Input: part model. Units: mm. Frame: model coordinates. Face numbers are marked on the shaded views. A direction names the side the tool comes from. Give positions to 0.01 mm unless a question says otherwise; leave off trailing zeros. Write each loop counter-clockwise with the first axis right and the second up, starting at its lowest first coordinate (ties: lowest second). Pieces come first, ordered by that corner, then holes. Notation, with made-up numbers: (4, -9.75) -> (57, -9.75) arc R35 cw to (57, 29.25) -> close; hole circle Ø3 at (1, 52.25). An arc over 180 degrees is marked (long way). Answer as a JSON object with one key per item and string values. Group by question number.
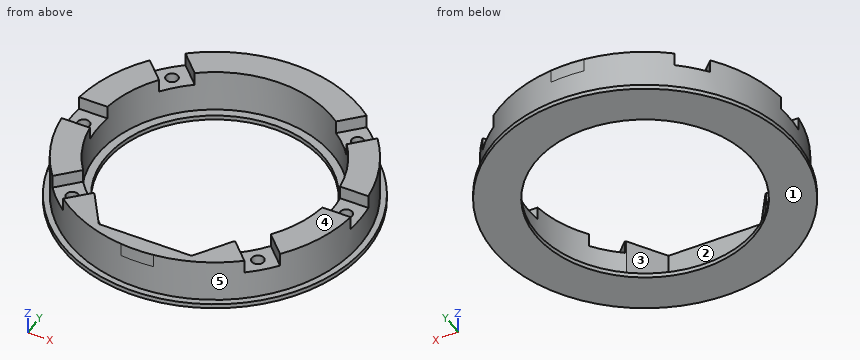
Autodesk Inventor part; units mm, degrees
ref_plane "YZ Plane" through (0, 0, 0) normal (1, 0, 0) x (0, 1, 0)
ref_plane "XZ Plane" through (0, 0, 0) normal (0, 1, 0) x (-1, 0, 0)
ref_plane "XY Plane" through (0, 0, 0) normal (0, 0, 1) x (1, 0, 0)
sketch "Skizze1" plane through (0, 0, 0) normal (0, 0, 1) x (1, 0, 0)
  circle A0 centre (0, 0) radius 18
  circle A1 centre (0, 0) radius 25
  dimension "d0" = 36
  dimension "d1" = 50
extrude "Extrusion1" add sketch "Skizze1" along normal blind 35
sketch "Skizze2" plane through (0, 0, 35) normal (0, 0, 1) x (1, 0, 0)
  circle A0 centre (0, 0) radius 19.3
  line L0 (0, -19.3) -> (0, -21.4)
  line L1 (0, -21.4) -> (-7.65, -21.4)
  line L2 (-7.65, -21.4) -> (7.65, -21.4)
  line L3 (7.65, -21.4) -> (7.65, -17.7191)
  line L4 (-7.65, -21.4) -> (-7.65, -17.7191)
  circle A1 centre (0, 0) radius 25
  circle A2 centre (0, 0) radius 18
  circle A3 centre (0, 0) radius 25
  circle A4 centre (0, 0) radius 18
  circle A5 centre (0, 0) radius 19.3
  dimension "d4" = 38.6
  dimension "d5" = 2.1
  dimension "d6" = 7.65
  dimension "d7" = 90
  dimension "d8" = 15.3
extrude "Extrusion2" cut sketch "Skizze2" against normal blind 34 contours A0 | A0 L0 L1 L4 | L3 L2 L0 A0 | A2
fillet "Rundung1" radius 4 2 edges at (-7.65, -17.7191, 18) (7.65, -17.7191, 18)
sketch "Skizze3" plane through (0, 0, 35) normal (0, 0, 1) x (1, 0, 0)
  arc A0 (9.65, -16.7143) -> (7.65, -20.1784) centre (11.65, -20.1784) ccw
  line L0 (7.65, -20.1784) -> (7.65, -21.4)
  line L1 (7.65, -21.4) -> (-7.65, -21.4)
  line L2 (-7.65, -21.4) -> (-7.65, -20.1784)
  arc A1 (-7.65, -20.1784) -> (-9.65, -16.7143) centre (-11.65, -20.1784) ccw
  arc A2 (9.65, -16.7143) -> (-9.65, -16.7143) centre (0, 0) ccw
  circle A3 centre (0, 0) radius 25
extrude "Extrusion3" cut sketch "Skizze3" against normal blind 25
sketch "Skizze4" plane through (0, 0, 10) normal (0, 0, 1) x (1, 0, 0)
  circle A0 centre (0, 0) radius 24
  circle A1 centre (0, 0) radius 25
  arc A2 (9.65, -16.7143) -> (7.65, -20.1784) centre (11.65, -20.1784) ccw
  line L0 (7.65, -21.4) -> (7.65, -20.1784)
  line L1 (-7.65, -21.4) -> (7.65, -21.4)
  line L2 (-7.65, -20.1784) -> (-7.65, -21.4)
  arc A3 (-7.65, -20.1784) -> (-9.65, -16.7143) centre (-11.65, -20.1784) ccw
  arc A4 (9.65, -16.7143) -> (-9.65, -16.7143) centre (0, 0) ccw
  dimension "d14" = 48
extrude "Extrusion4" cut sketch "Skizze4" against normal blind 9.25 contours A1
sketch "Skizze5" plane through (0, 0, 10) normal (0, 0, 1) x (1, 0, 0)
  circle A0 centre (0, 0) radius 24
  arc A1 (9.65, -16.7143) -> (7.65, -20.1784) centre (11.65, -20.1784) ccw
  line L0 (7.65, -21.4) -> (7.65, -20.1784)
  line L1 (-7.65, -21.4) -> (7.65, -21.4)
  line L2 (-7.65, -20.1784) -> (-7.65, -21.4)
  arc A2 (-7.65, -20.1784) -> (-9.65, -16.7143) centre (-11.65, -20.1784) ccw
  arc A3 (9.65, -16.7143) -> (-9.65, -16.7143) centre (0, 0) ccw
extrude "Extrusion5" cut sketch "Skizze5" against normal blind 2.2
sketch "Skizze6" plane through (0, 0, 7.8) normal (0, 0, 1) x (1, 0, 0)
  line L0 (30, -2.706) -> (-30, -2.706)
  line L1 (-30, -2.706) -> (-30, 2.706)
  line L2 (-30, 2.706) -> (30, 2.706)
  line L3 (30, 2.706) -> (30, -2.706)
  line L4 (30, -2.706) -> (-30, 2.706) construction
  line L5 (-30, -2.706) -> (30, 2.706) construction
  point P0 (0, 0)
  dimension "d33" = 60
extrude "Extrusion6" cut sketch "Skizze6" against normal blind 2.2
sketch "Skizze7" plane through (0, 0, 5.6) normal (0, 0, 1) x (1, 0, 0)
  line L0 (-22.5614, -2.035) -> (-22.5614, 2.035)
  line L1 (-22.5614, 0) -> (-19.3, 0)
  arc A0 (-19.1094, 2.706) -> (-19.1094, -2.706) centre (0, 0) ccw
  line L2 (-19.3, 0) -> (-24, 0)
  circle A1 centre (0, 0) radius 24
  circle A2 centre (-21.65, 0) radius 0.9
  dimension "d34" = 1.8
extrude "Extrusion7" cut sketch "Skizze7" against normal blind 4 contours A2 L1 | L1 A2
mirror "Spiegeln1" about plane through (0, 0, 0) normal (1, 0, 0) of "Extrusion7"
sketch "Skizze8" plane through (0, 0, 7.8) normal (0, 0, 1) x (1, 0, 0)
  point P0 (0, 0)
pattern_circular "Runde Anordnung1" count 8 over 360 about axis through (0, 0, -10) along (0, 0, 1) of "Extrusion7", "Extrusion6"
sketch "Skizze9" plane through (0, -20.9307, 1.6) normal (0, 0, 1) x (1, 0, 0)
  line L0 (-0.8646, -0.4693) -> (0.8646, -0.4693)
  line L1 (-2.706, -0.4693) -> (-0.8646, -0.4693)
  line L2 (-2.706, 40.0401) -> (-2.706, 44.7777)
  line L3 (2.706, 44.7777) -> (2.706, 40.0401)
  arc A0 (2.706, 44.7777) -> (-2.706, 44.7777) centre (0, 20.9307) ccw
  arc A1 (2.706, 40.0401) -> (-2.706, 40.0401) centre (0, 20.9307) ccw
  arc A2 (-2.706, -2.9163) -> (2.706, -2.9163) centre (0, 20.9307) ccw
  line L4 (2.706, -0.4693) -> (2.706, -2.9163)
  line L5 (-2.706, -2.9163) -> (-2.706, -0.4693)
  line L6 (0.8646, -0.4693) -> (2.706, -0.4693)
  arc A3 (-0.8646, -0.4693) -> (0.8646, -0.4693) centre (0, -0.7193) ccw
  arc A4 (-0.8646, -0.4693) -> (0.8646, -0.4693) centre (0, -0.7193) ccw
extrude "Extrusion8" add sketch "Skizze9" along normal blind 4 contours L0 A3
sketch "Skizze10" plane through (-2.706, -21.4, 5.6) normal (0, 0, 1) x (1, 0, 0)
  line L0 (0, 0) -> (5.412, 0)
  line L1 (0, 40.5094) -> (0, 45.247)
  line L2 (5.412, 45.247) -> (5.412, 40.5094)
  arc A0 (5.412, 45.247) -> (0, 45.247) centre (2.706, 21.4) ccw
  arc A1 (5.412, 40.5094) -> (0, 40.5094) centre (2.706, 21.4) ccw
  arc A2 (0, -2.447) -> (5.412, -2.447) centre (2.706, 21.4) ccw
  line L3 (5.412, 0) -> (5.412, -2.447)
  line L4 (0, -2.447) -> (0, 0)
extrude "Extrusion9" add sketch "Skizze10" along normal up to surface (2.2 mm away)
sketch "Skizze11" plane through (0, 0, 7.8) normal (0, 0, 1) x (-0.3826834, -0.9238795, 0)
  line L0 (15.7149, 14.7896) -> (16.8435, 15.2571)
  arc A0 (11.7491, 15.3117) -> (9.8128, 16.6192) centre (0, 0) ccw
  line L1 (16.8435, 15.2571) -> (11.7491, 15.3117)
  line L2 (-18.6903, 4.8128) -> (-23.0673, 6.6258)
  arc A1 (9.8128, -16.6192) -> (16.6192, -9.8128) centre (0, 0) ccw
  line L3 (9.8128, -16.6192) -> (11.6258, -20.9962)
  line L4 (6.6258, -23.0673) -> (4.8128, -18.6903)
  arc A2 (-4.8128, -18.6903) -> (4.8128, -18.6903) centre (0, 0) ccw
  line L5 (-4.8128, -18.6903) -> (-6.6258, -23.0673)
  line L6 (4.8128, 18.6903) -> (6.6258, 23.0673)
  line L7 (20.9962, -11.6258) -> (16.6192, -9.8128)
  line L8 (18.6903, -4.8128) -> (23.0673, -6.6258)
  arc A3 (-9.8128, 16.6192) -> (-16.6192, 9.8128) centre (0, 0) ccw
  line L9 (-9.8128, 16.6192) -> (-11.6258, 20.9962)
  line L10 (-6.6258, 23.0673) -> (-4.8128, 18.6903)
  arc A4 (4.8128, 18.6903) -> (-4.8128, 18.6903) centre (0, 0) ccw
  line L11 (-11.6258, -20.9962) -> (-9.8128, -16.6192)
  line L12 (11.6258, 20.9962) -> (9.8128, 16.6192)
  arc A5 (11.7491, 15.3117) -> (9.8128, 16.6192) centre (0, 0) ccw
  arc A6 (11.7491, 15.3117) -> (15.7149, 14.7896) centre (14.1841, 18.4851) ccw
  line L13 (16.8435, 15.2571) -> (15.7149, 14.7896)
  line L14 (22.6986, 1.1217) -> (16.8435, 15.2571)
  line L15 (21.5699, 0.6543) -> (22.6986, 1.1217)
  arc A7 (21.5699, 0.6543) -> (19.1349, -2.5192) centre (23.1007, -3.0413) ccw
  arc A8 (18.6903, -4.8128) -> (19.1349, -2.5192) centre (0, 0) ccw
  line L16 (-20.9962, 11.6258) -> (-16.6192, 9.8128)
  arc A9 (-6.6258, -23.0673) -> (6.6258, -23.0673) centre (0, 0) ccw
  arc A10 (-18.6903, 4.8128) -> (-9.8128, -16.6192) centre (0, 0) ccw
  arc A11 (-23.0673, 6.6258) -> (-11.6258, -20.9962) centre (0, 0) ccw
  arc A12 (-11.6258, 20.9962) -> (-20.9962, 11.6258) centre (0, 0) ccw
  arc A13 (11.6258, -20.9962) -> (20.9962, -11.6258) centre (0, 0) ccw
  arc A14 (6.6258, 23.0673) -> (-6.6258, 23.0673) centre (0, 0) ccw
  arc A15 (23.0673, -6.6258) -> (11.6258, 20.9962) centre (0, 0) ccw
  point P0 (15.7149, 14.7896)
extrude "Extrusion10" cut sketch "Skizze11" against normal up to surface (6.8 mm away) contours A6 L1 L0
mirror "Spiegeln2" about plane through (0, 0, 0) normal (1, 0, 0) of "Extrusion10"
sketch "Skizze12" plane through (0, 0, 7.8) normal (0, 0, 1) x (-0.3826834, -0.9238795, 0)
  point P0 (0, 0)
sketch "Skizze13" plane through (0, 0, 7.8) normal (0, 0, 1) x (1, 0, 0)
  line L0 (-7.65, -21.4) -> (-9.65, -16.7143)
  arc A0 (-11.5989, -15.4258) -> (-9.65, -16.7143) centre (0, 0) ccw
  line L1 (-11.5989, -15.4258) -> (-14.9489, -18.7758)
  arc A1 (-14.9489, -18.7758) -> (14.9489, -18.7758) centre (0, 0) ccw
  line L2 (14.9489, -18.7758) -> (11.5989, -15.4258)
  arc A2 (9.65, -16.7143) -> (11.5989, -15.4258) centre (0, 0) ccw
  line L3 (9.65, -16.7143) -> (7.65, -21.4)
  line L4 (-7.65, -21.4) -> (7.65, -21.4)
  arc A3 (-11.5989, -15.4258) -> (-9.65, -16.7143) centre (0, 0) ccw
  line L5 (7.65, -21.4) -> (-7.65, -21.4)
  line L6 (-11.5989, -15.4258) -> (-7.65, -21.4)
extrude "Extrusion11" cut sketch "Skizze13" against normal up to surface (6.8 mm away) contours L6 A0 L0
mirror "Spiegeln3" about plane through (0, 0, 0) normal (1, 0, 0) of "Extrusion11"
sketch "Skizze14" plane through (0, 0, 1) normal (0, 0, 1) x (1, 0, 0)
  point P0 (0, 0)
sketch "Skizze15" plane through (0, 0, 7.8) normal (0, 0, 1) x (1, 0, 0)
  circle A0 centre (0, 0) radius 19.375
  dimension "d37" = 38.75
extrude "Extrusion12" cut sketch "Skizze15" against normal up to surface (7.05 mm away)
sketch "Skizze16" plane through (0, 0, 7.8) normal (0, 0, 1) x (1, 0, 0)
  circle A0 centre (-15.3089, 15.3089) radius 0.9
  circle A1 centre (-15.3089, 15.3089) radius 1
  circle A2 centre (-21.65, 0) radius 0.9
  circle A3 centre (-21.65, 0) radius 1
  circle A4 centre (-15.3089, -15.3089) radius 0.9
  circle A5 centre (-15.3089, -15.3089) radius 1
  circle A6 centre (15.3089, -15.3089) radius 0.9
  circle A7 centre (15.3089, -15.3089) radius 1
  circle A8 centre (21.65, 0) radius 0.9
  circle A9 centre (21.65, 0) radius 1
  circle A10 centre (15.3089, 15.3089) radius 0.9
  circle A11 centre (15.3089, 15.3089) radius 1
  point P0 (0, 0)
  dimension "d40" = 2
  dimension "d41" = 2
  dimension "d42" = 2
  dimension "d43" = 2
  dimension "d44" = 2
  dimension "d45" = 2
extrude "Extrusion13" cut sketch "Skizze16" against normal up to surface (7.05 mm away) contours A0 | A1 | A2 | A3 | A4 | A5 | A7 | A8 | A9 | A11
properties part number "LCDmount_3D-Druck"
1. Reachability of the marked faces 1 and 2 from +Z, -Z, +X, -X, +Y, -Y: full face, straight path, thin tool, end or side. Return the list, or none.
2. Mould query, pull axis Y, two halves, no side actions, for the marked faces 3, 4 and 5. Classes: pulls with the +Y half, pulls with the -Y half, needs draft (parallel to the pull), parting line crosses it, or undercut.
3. Section A-A (z = 6.5). Return the cut outline in (x, y) (3 decimals).
4. Line query: line 1 (Y direction, x = 0, z = 0.6); line 2 (X direction, y = -16, z = 4.75); line 3 (X direction, y = 17.5, z = 3). Output: solid intervals per line, ascending.
5. Section B-B (x = 0). Return the cut outline in (y, z) (3 decimals), plus the area to 3 significant figures.
6. Section D-D (x = -6). Return the cut outline in (y, z), plus the area to 3 significant figures.
7. Contact query for flat-ended pins moving along their axis: pin 1 Ø1.1 at (x, z) = (-22, 7) entering from +Y; pin 2 Ø0.7 at (x, z) = (22.5, 6.5) entering from -Y; pin 3 Ø15 at (x, y) = (12, 2.5) entering from +Z; pin 4 Ø0.7 at (x, z) = (-22, 6.5) entering from -Y. Output: stop coordinate, or through.
8. Section C-C (y = 0). Return the cut outline in (x, z) (3 decimals), plus the area to 3 significant figures.
Working result:
{
 "1": {"face 1": "-Z, +X, -X, +Y, -Y", "face 2": "+Z"},
 "2": {"face 3": "undercut", "face 4": "needs draft", "face 5": "parting line crosses it"},
 "3": {"outline": "(-23.847, -2.706) arc R24 ccw to (-18.776, -14.949) -> (-15.479, -11.652) arc R19.375 cw to (-19.185, -2.706) -> close; (-23.847, 2.706) -> (-19.185, 2.706) arc R19.375 cw to (-15.479, 11.652) -> (-18.776, 14.949) arc R24 ccw to start; (-14.949, -18.776) arc R24 ccw to (14.949, -18.776) -> (11.652, -15.479) arc R19.375 cw to (11.477, -15.61) -> (7.65, -21.4) -> (-7.65, -21.4) -> (-11.477, -15.61) arc R19.375 cw to (-11.652, -15.479) -> close; (-14.949, 18.776) -> (-11.652, 15.479) arc R19.375 cw to (11.652, 15.479) -> (14.949, 18.776) arc R24 ccw to start; (15.479, -11.652) -> (18.776, -14.949) arc R24 ccw to (23.847, -2.706) -> (19.185, -2.706) arc R19.375 cw to start; (15.479, 11.652) arc R19.375 cw to (19.185, 2.706) -> (23.847, 2.706) arc R24 ccw to (18.776, 14.949) -> close"},
 "4": {"line 1": "y = -25 to -18, 18 to 25", "line 2": "x = -17.89 to -16.03, -14.59 to -11.22, 11.22 to 14.59, 16.03 to 17.89", "line 3": "x = -16.42 to -8.32, 8.32 to 16.42"},
 "5": {"outline": "(-25, 0) -> (-18, 0) -> (-18, 0.75) -> (-19.375, 0.75) -> (-19.375, 1) -> (-21.4, 1) -> (-21.4, 7.8) -> (-24, 7.8) -> (-24, 0.75) -> (-25, 0.75) -> close; (18, 0) -> (25, 0) -> (25, 0.75) -> (24, 0.75) -> (24, 7.8) -> (19.375, 7.8) -> (19.375, 0.75) -> (18, 0.75) -> close; hole (20.75, 1.6) -> (22.55, 1.6) -> (22.55, 5.6) -> (20.75, 5.6) -> close", "area": "54.7 mm^2"},
 "6": {"outline": "(-24.27, 0) -> (-16.97, 0) -> (-16.97, 0.75) -> (-18.42, 0.75) -> (-18.42, 1) -> (-21.4, 1) -> (-21.4, 7.8) -> (-23.24, 7.8) -> (-23.24, 0.75) -> (-24.27, 0.75) -> close; (16.97, 0) -> (24.27, 0) -> (24.27, 0.75) -> (23.24, 0.75) -> (23.24, 7.8) -> (18.42, 7.8) -> (18.42, 0.75) -> (16.97, 0.75) -> close", "area": "58.6 mm^2"},
 "7": {"pin 1": "stops at y = 10.77", "pin 2": "stops at y = -9.24", "pin 3": "stops at z = 7.8", "pin 4": "stops at y = -10.36"},
 "8": {"outline": "(-25, 0) -> (-18, 0) -> (-18, 0.75) -> (-19.375, 0.75) -> (-19.375, 5.6) -> (-20.65, 5.6) -> (-20.65, 0.75) -> (-22.65, 0.75) -> (-22.65, 5.6) -> (-24, 5.6) -> (-24, 0.75) -> (-25, 0.75) -> close; (18, 0) -> (25, 0) -> (25, 0.75) -> (24, 0.75) -> (24, 5.6) -> (22.65, 5.6) -> (22.65, 0.75) -> (20.65, 0.75) -> (20.65, 5.6) -> (19.375, 5.6) -> (19.375, 0.75) -> (18, 0.75) -> close", "area": "36.0 mm^2"}
}
